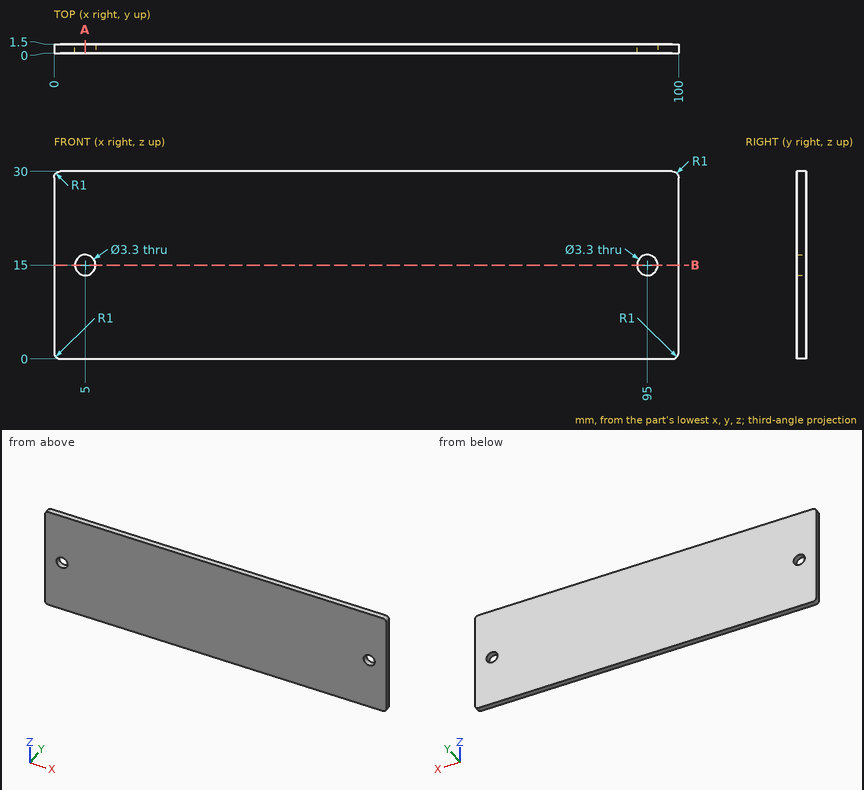
Print and shaded views of the part. All mm, measured from the part's lowest x, y and z. Round coordinates to 2 decimals unless told otherwise and drop trailing zeros. Write each loop counter-clockwise with the first axis right and the second up, starting at its lowest first coordinate (ties: lowest second). Pieces come first, ordered by that corner, then holes. Notation, with made-up numbers: M 32.25,7 L 65.25,7 A19 cw 65.25,20 Z; hole C 58,-15.75 d4. An arc over 180 degrees is marked long. Use a Markdown table: item, result. Add a question column.
1. Slice it at A-A on x = 5. Give the cut face in (y, z), then the cut area to 4 significant figures.
2. Drill centre lines: probe 1 along Z at (x, y) = (5, 0.7); probe 2 along X at (y, z) = (0.4, 13.5); probe 3 along X at (y, z) = (1.15, 15.5). Where is each one in solid material? Low to high.
3. Flat gauge pin, fed straight in: P1, Ø2, axis at x = 63, z = 10.5, coming from the -Y side. Where does the tip first touch, or does it go through?
4. Slice it at B-B on z = 15. Give the cut face in (x, y), then the cut area to 3 significant figures.
Reply:
| question | item | result |
|---|---|---|
| 1 | outline | M 0,0 L 1.5,0 L 1.5,13.35 L 0,13.35 Z; M 0,16.65 L 1.5,16.65 L 1.5,30 L 0,30 Z |
| 1 | area | 40.05 mm^2 |
| 2 | probe 1 | z = 0 to 13.35, 16.65 to 30 |
| 2 | probe 2 | x = 0 to 4.31, 5.69 to 94.31, 95.69 to 100 |
| 2 | probe 3 | x = 0 to 3.43, 6.57 to 93.43, 96.57 to 100 |
| 3 | P1 | stops at y = 0 |
| 4 | outline | M 0,0 L 3.35,0 L 3.35,1.5 L 0,1.5 Z; M 6.65,0 L 93.35,0 L 93.35,1.5 L 6.65,1.5 Z; M 96.65,0 L 100,0 L 100,1.5 L 96.65,1.5 Z |
| 4 | area | 140 mm^2 |
